from build123d import *

# Parameters (mm, degrees)
CROQUIS5_R            = 1.5
CORTAR_EXTRUIR3_DEPTH = 10


with BuildPart() as part:
    # Croquis3 → Revolución3 (revolve)
    with BuildSketch(Plane(origin=(0, 0, 0), x_dir=(1, 0, 0), z_dir=(0, 1, 0))):
        with BuildLine():
            Line((0, 3.75), (2.5, 3.75))
            Line((2.5, 3.75), (2, 2.466364983))
            Line((2, 2.466364983), (1.836579632, 2.046820768))
            ThreePointArc((1.836579632, 2.046820768), (2.75, 0), (1.836579632, -2.046820768))
            Line((1.836579632, -2.046820768), (2, -2.466364983))
            Line((2, -2.466364983), (2.5, -3.75))
            Line((2.5, -3.75), (0, -3.75))
            Line((0, -3.75), (0, 3.75))
        make_face()
    revolve(axis=Axis((0, 0, -3.75), (0, 0, 1)))

    # Croquis5 → Cortar-Extruir3 (cut)
    with BuildSketch(Plane(origin=(0, 0, -3.75), x_dir=(-1, 0, 0), z_dir=(0, 0, -1))):
        Circle(CROQUIS5_R)
    extrude(amount=-CORTAR_EXTRUIR3_DEPTH, mode=Mode.SUBTRACT)


solid = part.part
Design review of the part built by this model. Coordinates are the model's own, in mm. Give positions to 0.01 mm unless a question says otherwise; leave off trailing zeros. Write each loop counter-clockwise with the first axis right and the second up, starting at its lowest first coordinate (ties: lowest second). Pieces come first, ordered by that corner, then holes. Notation, with made-up numbers: M 41.25,63 L 83.25,63 A22 ccw 83.25,79 Z; hole C 39,-3.75 d11. An arc over 180 degrees is marked long. Return JSON: item names as keys, results as strings. Group by question number.
Item 1: Take a section at D-D (z = 1.75). Give the boundary of the cut face in (x, y).
Item 2: Take a section at A-A (x = 2.35). Count the separate pieces of the cut face and the enclosed holes in it, plus the area to 3 significant figures.
Item 3: The part is to be moulded in two halves that separate along X. For faces 1 (the cylindrical face through (1.5, 0.07, -0.05)), 2 (the flat face through (-2, 0, -3.75)), say which applies: pulls with the +X half, pulls with the -X half, needs draft (parallel to the pull), parting line crosses it, or undercut.
Item 4: Wall thickness on line 1 along Z through (x, y) = (-0.6, 2.2); line 2 along Z through (x, y) = (0.6, -1.8); line 3 along Y through (x, z) = (1.25, -2): over which ranges is each line inside the solid? List them lowest first.
Item 5: Take a section at B-B (z = 1). Give the boundary of the cut face in (x, y), plus the area to 3 significant figures.
Item 6: Clearance check with flat-ended pins moving along their axes: pin 1 Ø3 at (x, z) = (0, -2) entering from -Y; pin 2 Ø2 at (y, z) = (2, -2) entering from +X. State where each tip first meets the part, or that it passes through.
Return value:
{
 "1": {"outline": "C 0,0 d4.24; hole C 0,0 d3"},
 "2": {"separate pieces": "3", "enclosed holes": "0", "area": "7.28 mm2"},
 "3": {"face 1": "undercut", "face 2": "needs draft"},
 "4": {"line 1": "z = -3.75 to -3.19, -1.54 to 1.54, 3.19 to 3.75", "line 2": "z = -3.75 to -2.2, -1.99 to 1.99, 2.2 to 3.75", "line 3": "y = -1.41 to -0.83, 0.83 to 1.41"},
 "5": {"outline": "C 0,0 d5.12; hole C 0,0 d3", "area": "13.5 mm2"},
 "6": {"pin 1": "stops at y = -2.7", "pin 2": "stops at x = 2.05"}
}
